Here's the drawing with two shaded views (mm, measured from the low corner). I have some questions. Give positions to 0.01 mm unless a question says otherwise; leave off trailing zeros. Loops run counter-clockwise (first coordinate to the right, second up) from the corner with the lowest first, then second, coordinate; pieces in that order, holes last. Notation, with made-up numbers: M 18,-9.75 L 61,-9.75 A30 ccw 61,25.25 Z; hole C 38.25,13 d1. An arc over 180 degrees is marked long. Use CSV: the item, a comma, the result in double quotes.
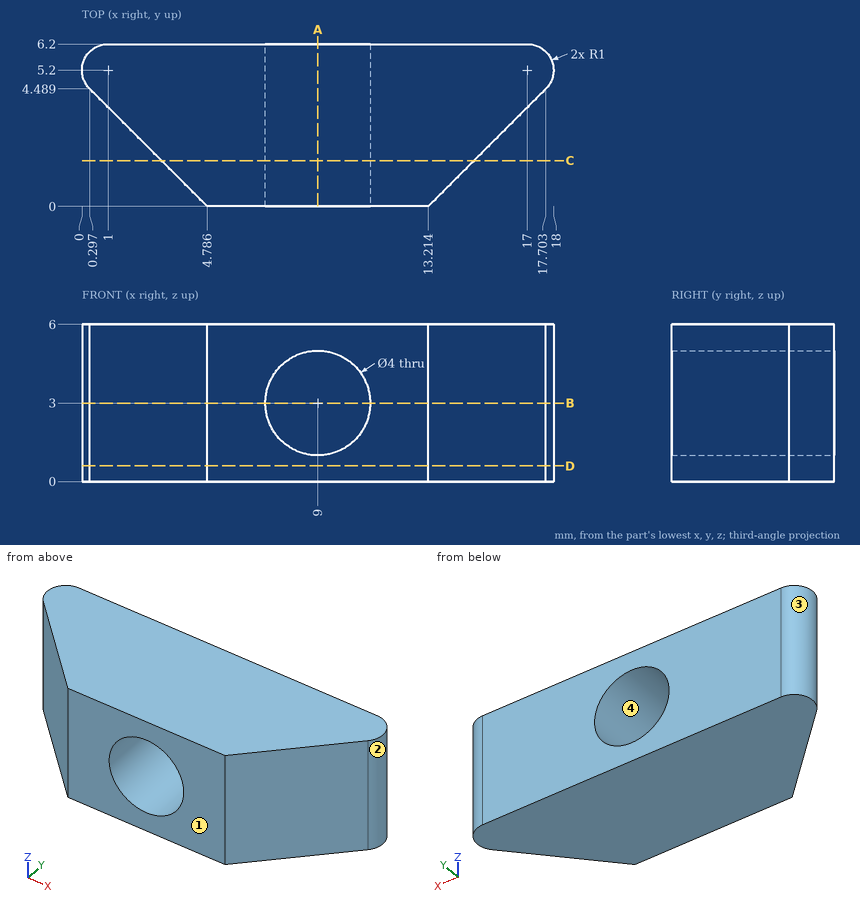
1. I want a section at C-C, the plane y = 1.75. List the corners of the cut face in (x, z) for me.
Outcome:
outline,"M 3.04,0 L 14.96,0 L 14.96,6 L 3.04,6 Z; hole C 9,3 d4"
2. I want a section at A-A, the plane x = 9. List the corners of the cut face in (y, z) for me.
Outcome:
outline,"M 0,0 L 6.2,0 L 6.2,1 L 0,1 Z; M 0,5 L 6.2,5 L 6.2,6 L 0,6 Z"
3. I want a section at D-D, the plane z = 0.6. List the corners of the cut face in (x, y) for me, then the cut area to 3 significant figures.
Outcome:
outline,"M 0.3,4.49 L 4.79,0 L 13.21,0 L 17.7,4.49 A1 ccw 17,6.2 L 1,6.2 A1 ccw Z"
area,"88.2 mm2"
4. I'm going to push a flat-ended pin straight in: pin 1 Ø2 at (y, z) = (2, 3.5) entering from -X (1 decimal). Where does the tip first touch, or does it pass through?
Outcome:
pin 1,"x = 1.8"
5. If we mould it in two halves opening along X, with no side actions, what happens to the marked faces 1, 2, 3 and 4? For each: +X half, -X half, draft (parallel to the pull), parting line (faces both ways), or undercut.
Outcome:
face 1,"draft"
face 2,"+X half"
face 3,"-X half"
face 4,"undercut"
6. I want a section at B-B, the plane z = 3. List the corners of the cut face in (x, y) for me.
Outcome:
outline,"M 0.3,4.49 L 4.79,0 L 7,0 L 7,6.2 L 1,6.2 A1 ccw Z; M 11,0 L 13.21,0 L 17.7,4.49 A1 ccw 17,6.2 L 11,6.2 Z"
7. Please list where these lines run through material, in increasing order: line 1 (Z direction, x = 9, y = 4.25); line 2 (X direction, y = 3.5, z = 3) (1 decimal); line 3 (X direction, y = 2, z = 3) (1 decimal).
Outcome:
line 1,"0 to 1, 5 to 6"
line 2,"1.3 to 7, 11 to 16.7"
line 3,"2.8 to 7, 11 to 15.2"
